from build123d import *

# Parameters (mm, degrees)
SKETCH_1_R          = 4.5
EXTRUDE_1_DEPTH     = 100
SKETCH_2_W          = 10.811132722
SKETCH_2_H          = 40
EXTRUDE_2_DEPTH     = 20
SKETCH_3_W          = 10.811132722
SKETCH_3_H          = 40
EXTRUDE_3_DEPTH     = 20
SKETCH_4_R          = 2.5
CUT_EXTRUDE_1_DEPTH = 11.811132722
SKETCH_5_R          = 4.25
CUT_EXTRUDE_2_DEPTH = 5
SKETCH_6_R          = 11
CUT_EXTRUDE_3_DEPTH = 7
SKETCH_7_R          = 11
CUT_EXTRUDE_4_DEPTH = 7


with BuildPart() as part:
    # Эскиз1 → Бобышка-Вытянуть1 (new body)
    with BuildSketch(Plane(origin=(0, 0, 0), x_dir=(0, 0, -1), z_dir=(1, 0, 0))):
        with BuildLine():
            Line((-24, 14.353267579), (-13.188867278, 14.353267579))
            Line((-13.188867278, 14.353267579), (-13.188867278, 11.502338019))
            ThreePointArc((-13.188867278, 11.502338019), (17.5, 0), (-13.188867278, -11.502338019))
            Line((-13.188867278, -11.502338019), (-13.188867278, -25.646732421))
            Line((-13.188867278, -25.646732421), (-24, -25.646732421))
            Line((-24, -25.646732421), (-24, 14.353267579))
        make_face()
        Circle(SKETCH_1_R, mode=Mode.SUBTRACT)
    extrude(amount=EXTRUDE_1_DEPTH)

    # Эскиз2 → Бобышка-Вытянуть2 (add)
    with BuildSketch(Plane.ZY):
        with Locations((18.594433639, -5.646732421)):
            Rectangle(SKETCH_2_W, SKETCH_2_H)
    extrude(amount=EXTRUDE_2_DEPTH)

    # Эскиз3 → Бобышка-Вытянуть3 (add)
    with BuildSketch(Plane(origin=(100, 0, 0), x_dir=(0, 0, -1), z_dir=(1, 0, 0))):
        with Locations((-18.594433639, -5.646732421)):
            Rectangle(SKETCH_3_W, SKETCH_3_H)
    extrude(amount=EXTRUDE_3_DEPTH)

    # Эскиз4 → Вырез-Вытянуть1 (cut, through all)
    with BuildSketch(Plane(origin=(0, 0, 13.188867278), x_dir=(-1, 0, 0), z_dir=(0, 0, -1))):
        with Locations((-110, 0)):
            Circle(SKETCH_4_R)
        with Locations((10, 0)):
            Circle(SKETCH_4_R)
    extrude(amount=-CUT_EXTRUDE_1_DEPTH, mode=Mode.SUBTRACT)

    # Эскиз5 → Вырез-Вытянуть2 (cut)
    with BuildSketch(Plane(origin=(0, 0, 13.188867278), x_dir=(-1, 0, 0), z_dir=(0, 0, -1))):
        with Locations((-110, 0)):
            Circle(SKETCH_5_R)
        with Locations((10, 0)):
            Circle(SKETCH_5_R)
    extrude(amount=-CUT_EXTRUDE_2_DEPTH, mode=Mode.SUBTRACT)

    # Эскиз6 → Вырез-Вытянуть3 (cut)
    with BuildSketch(Plane(origin=(100, 0, 0), x_dir=(0, 0, -1), z_dir=(1, 0, 0))):
        Circle(SKETCH_6_R)
    extrude(amount=-CUT_EXTRUDE_3_DEPTH, mode=Mode.SUBTRACT)

    # Эскиз7 → Вырез-Вытянуть4 (cut)
    with BuildSketch(Plane.ZY):
        Circle(SKETCH_7_R)
    extrude(amount=-CUT_EXTRUDE_4_DEPTH, mode=Mode.SUBTRACT)


solid = part.part
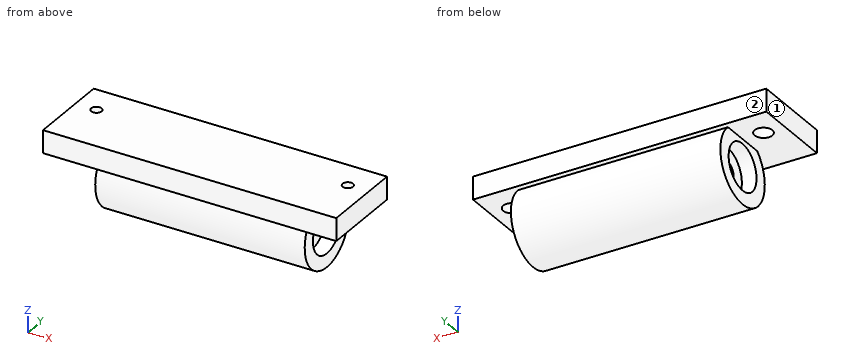
Work out the finished part from the listing and answer in its coordinate system (mm). Face numbers are marked on the shaded views. A direction names the side the tool comes from. Round coordinates to 2 decimals unless told otherwise and drop trailing zeros. Write each loop counter-clockwise with the first axis right and the second up, starting at its lowest first coordinate (ties: lowest second). Pieces come first, ordered by that corner, then holes.
1) Straight lines are drawn through the part: line 1 (Y direction, x = -10, z = 22); line 2 (Y direction, x = 3, z = 0); line 3 (X direction, y = -13, z = 3). For each, find the intervals that lie inside material, in ascending order.
2) A cutting plane is placed at B-B (x = 110). Give the vertices of the cut face in (y, z), plus the area to 3 significant figures.
3) A cutting plane is placed at A-A (z = 0). Give the vertices of the cut face in (x, y), plus the area to 3 significant figures.
4) A cutting plane is placed at C-C (z = 21). Give the vertices of the cut face in (x, y).
5) A tool of negligible diameter and unlimited length cuts with its end or side. For the marked faces 1 and 2, from which of +Z, -Z, +X, -X, +Y, -Y can it reach the whole face along a straight path? Write none if from no direction.
6) A cutting plane is placed at D-D (y = 0). Give the number of separate pieces and of enclosed holes in the cut face, plus the area to 3 significant figures.
7) Given pin 1 Ø13 at (y, z) = (0, 0) entering from +X; pin 2 Ø6.5 at (y, z) = (0.5, 0.5) entering from -X; pin 3 Ø4 at (x, z) = (88.5, 14.5) entering from +Y; pin 4 Ø24.5 at (y, z) = (3.5, -7) entering from -X, each flat-ended and moving along its own axis, determine where each tip first touches the part or whether it passes through.
Completed:
1. line 1: y = -25.65 to -2.5, 2.5 to 14.35
1. line 2: y = -17.5 to -11, 11 to 17.5
1. line 3: x = 0 to 100
2. outline: (-25.65, 13.19) - (-4.25, 13.19) - (-4.25, 18.19) - (-2.5, 18.19) - (-2.5, 24) - (-25.65, 24) - close; (2.5, 18.19) - (4.25, 18.19) - (4.25, 13.19) - (14.35, 13.19) - (14.35, 24) - (2.5, 24) - close
2. area: 361 mm2
3. outline: (0, -17.5) - (100, -17.5) - (100, -11) - (93, -11) - (93, -4.5) - (7, -4.5) - (7, -11) - (0, -11) - close; (0, 11) - (7, 11) - (7, 4.5) - (93, 4.5) - (93, 11) - (100, 11) - (100, 17.5) - (0, 17.5) - close
3. area: 2,420 mm2
4. outline: (-20, -25.65) - (120, -25.65) - (120, 14.35) - (-20, 14.35) - close; hole circle Ø5 at (-10, 0); hole circle Ø5 at (110, 0)
5. face 1: +Z, -Z, -X, +Y, -Y
5. face 2: +Z, +X, -X, +Y
6. separate pieces: 4
6. enclosed holes: 0
6. area: 3,360 mm2
7. pin 1: stops at x = 93
7. pin 2: passes through
7. pin 3: stops at y = 14.35
7. pin 4: stops at x = 0
